CAD build for the part. Positions are in the model's coordinates, mm. A direction names the side the tool comes from. Round coordinates to 2 decimals unless told otherwise and drop trailing zeros. Loops run counter-clockwise (first coordinate to the right, second up) from the corner with the lowest first, then second, coordinate; pieces in that order, holes last. Notation, with made-up numbers: M 21.25,2 L 33.25,2 A20 cw 33.25,24 Z; hole C -29.75,-4 d2. An arc over 180 degrees is marked long. One line per item, written item: value. Start each with the question number.
from build123d import *

# Parameters (mm, degrees)
SKETCH1_W                       = 50.8
SKETCH1_H                       = 50.8
BOSS_EXTRUDE1_DEPTH             = 9.525
F_1_2_0_5_DIAMETER_HOLE1_D      = 12.7
F_1_2_0_5_DIAMETER_HOLE1_DEPTH  = 70.104
F_1_2_0_5_DIAMETER_HOLE1_TIP    = 3.815464931
S_0_348_DIAMETER_HOLE1_D        = 8.8392
S_0_348_DIAMETER_HOLE1_DEPTH    = 70.104
S_0_348_DIAMETER_HOLE1_TIP      = 2.655563592
F_29_0_136_DIAMETER_HOLE1_D     = 3.4544
F_29_0_136_DIAMETER_HOLE1_DEPTH = 70.104
F_29_0_136_DIAMETER_HOLE1_TIP   = 1.037806461
F_10_32_TAPPED_HOLE1_D          = 4.0386
F_10_32_TAPPED_HOLE1_DEPTH      = 11.938
F_10_32_TAPPED_HOLE1_TIP        = 1.213317848


with BuildPart() as part:
    # Sketch1 → Boss-Extrude1 (new body)
    with BuildSketch(Plane(origin=(0, 0, 0), x_dir=(0, 0, -1), z_dir=(1, 0, 0))):
        Rectangle(SKETCH1_W, SKETCH1_H)
    extrude(amount=BOSS_EXTRUDE1_DEPTH)

    # 1/2 (0.5) Diameter Hole1
    with Locations(Plane(origin=(9.525, 0, 0), x_dir=(0, 0, -1), z_dir=(1, 0, 0))):
        with Locations((0, -13.97)):
            Hole(F_1_2_0_5_DIAMETER_HOLE1_D / 2, depth=F_1_2_0_5_DIAMETER_HOLE1_DEPTH)
            with Locations((0, 0, -(F_1_2_0_5_DIAMETER_HOLE1_DEPTH + F_1_2_0_5_DIAMETER_HOLE1_TIP / 2))):  # 118° drill point
                Cone(0, F_1_2_0_5_DIAMETER_HOLE1_D / 2, F_1_2_0_5_DIAMETER_HOLE1_TIP, mode=Mode.SUBTRACT)

    # S (0.348) Diameter Hole1
    with Locations(Plane(origin=(9.525, 0, 0), x_dir=(0, 0, -1), z_dir=(1, 0, 0))):
        with Locations((0, 12.2301)):
            Hole(S_0_348_DIAMETER_HOLE1_D / 2, depth=S_0_348_DIAMETER_HOLE1_DEPTH)
            with Locations((0, 0, -(S_0_348_DIAMETER_HOLE1_DEPTH + S_0_348_DIAMETER_HOLE1_TIP / 2))):  # 118° drill point
                Cone(0, S_0_348_DIAMETER_HOLE1_D / 2, S_0_348_DIAMETER_HOLE1_TIP, mode=Mode.SUBTRACT)

    # #29 (0.136) Diameter Hole1
    with Locations(Plane(origin=(9.525, 0, 0), x_dir=(0, 0, -1), z_dir=(1, 0, 0))):
        with Locations((21, 12.2301), (-21, 11.74145915)):
            Hole(F_29_0_136_DIAMETER_HOLE1_D / 2, depth=F_29_0_136_DIAMETER_HOLE1_DEPTH)
            with Locations((0, 0, -(F_29_0_136_DIAMETER_HOLE1_DEPTH + F_29_0_136_DIAMETER_HOLE1_TIP / 2))):  # 118° drill point
                Cone(0, F_29_0_136_DIAMETER_HOLE1_D / 2, F_29_0_136_DIAMETER_HOLE1_TIP, mode=Mode.SUBTRACT)

    # #10-32 Tapped Hole1
    with Locations(Plane(origin=(-0.669296778, 7.980106856, -25.4), x_dir=(-1, 0, 0), z_dir=(0, 0, -1))):
        with Locations((-5.431796778, -27.030106856), (-5.431796778, 11.069893144)):
            Hole(F_10_32_TAPPED_HOLE1_D / 2, depth=F_10_32_TAPPED_HOLE1_DEPTH)
            with Locations((0, 0, -(F_10_32_TAPPED_HOLE1_DEPTH + F_10_32_TAPPED_HOLE1_TIP / 2))):  # 118° drill point
                Cone(0, F_10_32_TAPPED_HOLE1_D / 2, F_10_32_TAPPED_HOLE1_TIP, mode=Mode.SUBTRACT)


solid = part.part
(1) Mould opens along Z. For faces 1 (the cylindrical face through (4.696, 13.943, -21.225)), 2 (the cylindrical face through (4.7, 16.61, -0.58)), 3 (the flat face through (5, 0, 25.4)), 4 (the flat face through (0, 0, 0)) say: pulls with the +Z half, pulls with the -Z half, needs draft (parallel to the pull), parting line crosses it, or undercut.
(2) Slice it at A-A, the plane y = -13.97. List the corners of the cut face in (x, z) (3 decimals).
(3) Slice it at C-C, the plane z = -21. Count the separate pieces of the cut face and the enclosed holes in it, and give its area (3 significant figures).
(4) Slice it at B-B, the plane z = 0. List the corners of the cut face in (x, y) (1 decimal).
(5) Slice it at D-D, the plane x = 8.25. List the corners of the cut face in (y, z), and give its area (3 significant figures).
(6) Probe L1, parallel to Y at x = 4.75, z = -21; L2, parallel to Y at x = 6.25, z = 0; L3, parallel to Y at x = 4.5, z = -18. List the from-to ranges inside material, lowest first.
(7) Flat gauge pin, fed straight in: P1, Ø3, axis at x = 4.76, y = 19.05, coming from the -Z side. Where does the tip first touch, or does it go through?
(8) Which spindle directions (+Z, -Z, +X, -X, +Y, -Y) get a long thin tool onto all of the face, cutting with end or side? Do faces 5 (the cylindrical face through (4.32, 17.08, -19.35)), 6 (the flat face through (5, 0, -25.4)). Say none if no direction does.
Check result:
1. face 1: undercut
1. face 2: undercut
1. face 3: pulls with the +Z half
1. face 4: needs draft
2. outline: M 0,-25.4 L 9.525,-25.4 L 9.525,-6.35 L 0,-6.35 Z; M 0,6.35 L 9.525,6.35 L 9.525,25.4 L 0,25.4 Z
3. separate pieces: 2
3. enclosed holes: 2
3. area: 425 mm^2
4. outline: M 0,-25.4 L 9.5,-25.4 L 9.5,-20.3 L 0,-20.3 Z; M 0,-7.6 L 9.5,-7.6 L 9.5,7.8 L 0,7.8 Z; M 0,16.6 L 9.5,16.6 L 9.5,25.4 L 0,25.4 Z
5. outline: M -25.4,-25.4 L 25.4,-25.4 L 25.4,25.4 L -25.4,25.4 Z; hole C -13.97,0 d12.7; hole C 12.23,0 d8.84; hole C 11.74,21 d3.45; hole C 12.23,-21 d3.45
5. area: 2,370 mm^2
6. L1: y = -25.4 to -21.07, -17.03 to 10.5, 13.96 to 17.03, 21.07 to 25.4
6. L2: y = -25.4 to -20.32, -7.62 to 7.81, 16.65 to 25.4
6. L3: y = -25.4 to -21.05, -17.05 to 17.05, 21.05 to 25.4
7. P1: stops at z = -13.15
8. face 5: -Z
8. face 6: -Z, +X, -X, +Y, -Y
